Here's how the part is built. I have some questions about the finished solid (model axes, mm). A direction names the side the tool comes from. Round coordinates to 2 decimals unless told otherwise and drop trailing zeros. Order: outer loops, then holes, each group sorted by start corner. A loop starts at its lowest first (then second) coordinate and runs counter-clockwise, first axis right, second up. Notation, with made-up numbers: (-23, -12) -> (19, -12) arc R19 cw to (19, 8) -> close; hole circle Ø5 at (68, 86). An arc over 180 degrees is marked (long way). Use a Markdown table: item, result. Add a question column.
(1) I'm going to push flat-ended pins straight in: P1, Ø0.6, axis at y = 0, z = -9.5, coming from the +X side; P2, Ø1.6, axis at x = 4, y = 0, coming from the +Z side; P3, Ø0.9, axis at x = -0.5, y = -2.5, coming from the -Z side. Where does each tip first touch, or does it pass through?
(2) I want a section at B-B, the plane z = 2.5. Please give me the cut outline in (x, y), then the cut area to 3 significant figures.
(3) I want a section at D-D, the plane x = -7.75. Please give me the cut outline in (y, z), then the cut area to 3 significant figures.
(4) On a 3-axis mill with a long thin cutter (end or side, diameter ignored), from which of +Z, -Z, +X, -X, +Y, -Y can I reach the whole of each face in a straight line? I mean faces 5 (the face through (7.35, 0, -7)), 6 (the face through (1.5, -4, 1)), 7 (the face through (0, -3, 0)), 8 (the face through (-7.35, 0, -7)). Say none if no direction works.
(5) If I drill on probe 1 along Z at (x, y) = (-0.35, -1.85); probe 2 along Y at (x, z) = (3, -7.5); probe 3 along Z at (x, y) = (-2.75, -0.6), over which ranges is the centre line in solid material (lowest first)?
(6) Thinking about a two-plate mould opening in Y: for faces 1 (the face through (8, -0.65, -7)), 2 (the face through (-0.021, -1.416, 0.548)), 3 (the face through (0, -1.35, -7)), 4 (the face through (-1.5, 0, 1)), which applies, pulls with the +Y half, pulls with the -Y half, needs draft (parallel to the pull), parting line crosses it, or undercut?
(7) I want a section at A-A, the plane y = -1.85. Please give me the cut outline in (x, z), then the cut area to 3 significant figures.
(8) I want a section at C-C, the plane z = -1.5. Please give me the cut outline in (x, y), then the cut area to 3 significant figures.
from build123d import *

# Parameters (mm, degrees)
BOSS_EXTRUDE1_DEPTH = 15
SKETCH2_W           = 3
SKETCH2_H           = 1.5
SKETCH2_W_2         = 1.5
SKETCH2_H_2         = 2
BOSS_EXTRUDE3_DEPTH = 5
SKETCH4_R           = 2
CUT_EXTRUDE1_DEPTH  = 3


with BuildPart() as part:
    # Sketch1 → Boss-Extrude1 (new body)
    with BuildSketch(Plane.XY):
        Polygon((7.5, -0.65), (9.35, -0.65), (9.35, -1.35), (-9.35, -1.35), (-9.35, -0.65), (-7.5, -0.65), (-7.35, -0.65), (-7.35, -0.5), (-7.35, 0.35), (-7.35, 0.65), (7.35, 0.65), (7.35, 0.35), (7.35, -0.5), (7.35, -0.65), align=None)
    extrude(amount=-BOSS_EXTRUDE1_DEPTH)

    # Sketch2 → Boss-Extrude3 (add)
    with BuildSketch(Plane.XY):
        with Locations((0, -3.6)):
            Rectangle(SKETCH2_W, SKETCH2_H)
        Polygon((1.5, -1.35), (0, -1.35), (-1.5, -1.35), (-1.5, -2.85), (1.5, -2.85), align=None)
        with Locations((-0.75, -0.35)):
            Rectangle(SKETCH2_W_2, SKETCH2_H_2)
        with Locations((0.75, -0.35)):
            Rectangle(SKETCH2_W_2, SKETCH2_H_2)
    extrude(amount=BOSS_EXTRUDE3_DEPTH)

    # Sketch4 → Cut-Extrude1 (cut)
    with BuildSketch(Plane.ZY.offset(1.5)):
        with Locations(Location((2.5, -1.85, 0), (0, 0, 270))):
            Circle(SKETCH4_R)
    extrude(amount=-CUT_EXTRUDE1_DEPTH, mode=Mode.SUBTRACT)


solid = part.part
Taken from the geometry:
| question | item | result |
|---|---|---|
| 1 | P1 | stops at x = 7.35 |
| 1 | P2 | stops at z = 0 |
| 1 | P3 | stops at z = 0 |
| 2 | outline | (-1.5, -4.35) -> (1.5, -4.35) -> (1.5, -3.85) -> (-1.5, -3.85) -> close; (-1.5, 0.15) -> (1.5, 0.15) -> (1.5, 0.65) -> (-1.5, 0.65) -> close |
| 2 | area | 3.00 mm2 |
| 3 | outline | (-1.35, -15) -> (-0.65, -15) -> (-0.65, 0) -> (-1.35, 0) -> close |
| 3 | area | 10.5 mm2 |
| 4 | face 5 | +Z, -Z, +X, +Y |
| 4 | face 6 | +Z, +X, +Y, -Y |
| 4 | face 7 | -Z, +X, -X, -Y |
| 4 | face 8 | +Z, -Z, -X, +Y |
| 5 | probe 1 | z = 0 to 0.5, 4.5 to 5 |
| 5 | probe 2 | y = -1.35 to 0.65 |
| 5 | probe 3 | z = -15 to 0 |
| 6 | face 1 | pulls with the +Y half |
| 6 | face 2 | undercut |
| 6 | face 3 | pulls with the -Y half |
| 6 | face 4 | needs draft |
| 7 | outline | (-1.5, 0) -> (1.5, 0) -> (1.5, 0.5) -> (-1.5, 0.5) -> close; (-1.5, 4.5) -> (1.5, 4.5) -> (1.5, 5) -> (-1.5, 5) -> close |
| 7 | area | 3.00 mm2 |
| 8 | outline | (-9.35, -1.35) -> (9.35, -1.35) -> (9.35, -0.65) -> (7.35, -0.65) -> (7.35, 0.65) -> (-7.35, 0.65) -> (-7.35, -0.65) -> (-9.35, -0.65) -> close |
| 8 | area | 32.2 mm2 |
